from build123d import *

# Parameters (mm, degrees)
SKETCH1_W             = 4.5
SKETCH1_H             = 4.5
BOSS_EXTRUDE1_DEPTH   = 12
BOSS_EXTRUDE1_2_DEPTH = 12
SKETCH2_R             = 0.691748062
BOSS_EXTRUDE2_DEPTH   = 2
SKETCH3_W             = 12.5
SKETCH3_H             = 6.3
BOSS_EXTRUDE3_DEPTH   = 8
SKETCH4_R             = 2.715
BOSS_EXTRUDE4_DEPTH   = 16.5
SKETCH5_R             = 2.715
BOSS_EXTRUDE5_DEPTH   = 10.5
BOSS_EXTRUDE5_TAPER   = 4
SKETCH8_W             = 8
SKETCH8_H             = 19.014368052
BOSS_EXTRUDE8_DEPTH   = 4
BOSS_EXTRUDE8_TAPER   = 15
PROFILE1_R            = 1.3


with BuildPart() as part:
    # Sketch1 → Boss-Extrude1 (new body)
    with BuildSketch(Plane.XY):
        with Locations((3.245938438, 2.25)):
            Rectangle(SKETCH1_W, SKETCH1_H)
    extrude(amount=-BOSS_EXTRUDE1_DEPTH)



with BuildPart() as body_2:
    # Sketch1 → Boss-Extrude1 2 (new body)
    with BuildSketch(Plane.XY):
        with Locations((-3.254061562, 2.25)):
            Rectangle(SKETCH1_W, SKETCH1_H)
    extrude(amount=-BOSS_EXTRUDE1_2_DEPTH)


with BuildPart() as part_1:
    add(part.part)

    add(body_2.part)  # Boss-Extrude2 merges body 2
    # Sketch2 → Boss-Extrude2 (add)
    with BuildSketch(Plane(origin=(0, 0, -12), x_dir=(-1, 0, 0), z_dir=(0, 0, -1))):
        with Locations((3.25, 2.25)):
            Circle(SKETCH2_R)
        with Locations((-3.25, 2.25)):
            Circle(SKETCH2_R)
    extrude(amount=BOSS_EXTRUDE2_DEPTH)

    # Sketch3 → Boss-Extrude3 (add)
    with BuildSketch(Plane.XY):
        with Locations((0, 2.15)):
            Rectangle(SKETCH3_W, SKETCH3_H)
    extrude(amount=BOSS_EXTRUDE3_DEPTH)

    # Sketch4 → Boss-Extrude4 (add)
    with BuildSketch(Plane.XY.offset(8)):
        with Locations((3.25, 2.25)):
            Circle(SKETCH4_R)
        with Locations((-3.25, 2.25)):
            Circle(SKETCH4_R)
    extrude(amount=BOSS_EXTRUDE4_DEPTH)

    # Sketch5 → Boss-Extrude5 (add)
    with BuildSketch(Plane.XY.offset(24.5)):
        with Locations((-3.25, 2.25)):
            Circle(SKETCH5_R)
        with Locations((3.25, 2.25)):
            Circle(SKETCH5_R)
    extrude(amount=BOSS_EXTRUDE5_DEPTH, taper=BOSS_EXTRUDE5_TAPER)

    # Sketch8 → Boss-Extrude8 (add)
    with BuildSketch(Plane(origin=(0, 5.3, 0), x_dir=(1, 0, 0), z_dir=(0, 1, 0))):
        with Locations((0, 1.507184026)):
            Rectangle(SKETCH8_W, SKETCH8_H)
    extrude(amount=BOSS_EXTRUDE8_DEPTH, taper=BOSS_EXTRUDE8_TAPER)

    # Sweep1: sweep along a path in path1
    with BuildLine(Plane.XZ.offset(-2.25)) as sweep1_path:
        ThreePointArc((0, 35), (25, 60), (50, 35))
    # profile1 → Sweep1 (sweep)
    with BuildSketch(Plane.XY.offset(35)):
        with Locations((-3.25, 2.25)):
            Circle(PROFILE1_R)
        with Locations((3.25, 2.25)):
            Circle(PROFILE1_R)
    sweep(path=sweep1_path.line)


solid = part_1.part
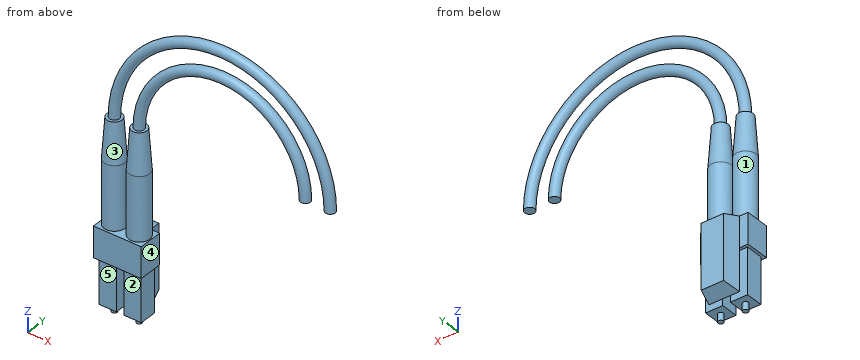
CAD build for the part. Positions are in the model's coordinates, mm. Face numbers are marked on the shaded views. A direction names the side the tool comes from. Round coordinates to 2 decimals unless told otherwise and drop trailing zeros. Loops run counter-clockwise (first coordinate to the right, second up) from the corner with the lowest first, then second, coordinate; pieces in that order, holes last.
(1) Wall check: line 1 along X through (y, z) = (2.5, 54); line 2 along X through (y, z) = (2.75, 40.5); line 3 along X through (y, z) = (0, 20). Give the ranges that are in metal, low to high.
(2) Which spindle directions (+Z, -Z, +X, -X, +Y, -Y) get a long thin tool onto all of the face, cutting with end or side? Do the marked faces 3, 4 and 5. Say none if no direction does.
(3) Cut at B-B (z = -1). State how many separate pieces and enclosed holes the cut face has, plus the area to 3 significant figures.
(4) Drop flat-ended pins along their axis: pin 1 (3 mm diameter, centred on y = 2.5, z = 2.5, fed in from +X); pin 2 (2 mm diameter, centred on y = 1, z = 47, fed in from -X); pin 3 (3 mm diameter, centred on x = 4, y = 2, fed in from +Z). Give the stop position or say it passes through.
(5) Two-plate mould, pull along Z, no slides. Class the marked faces 1 and 2: +Z half, -Z half, draft (parallel to the pull), parting line (faces both ways), or undercut.
(6) Cut at A-A (z = 9.5). Give the cut face in (x, y) (3 decimals).
Findings below:
1. line 1: x = 2.4 to 5.85, 11.99 to 17.37, 32.63 to 38.01, 44.15 to 47.6
1. line 2: x = -3.93 to -1.48, 2.72 to 5.2, 44.8 to 47.28, 51.48 to 53.93
1. line 3: x = -4.77 to -1.73, 1.73 to 4.77
2. face 3: none
2. face 4: -Z, +X, +Y, -Y
2. face 5: -Z, +X, -X, -Y
3. separate pieces: 3
3. enclosed holes: 0
3. area: 68.2 mm2
4. pin 1: stops at x = 6.25
4. pin 2: stops at x = -2.18
4. pin 3: stops at z = 57.19
5. face 1: undercut
5. face 2: draft
6. outline: circle Ø5.43 at (-3.25, 2.25); circle Ø5.43 at (3.25, 2.25)
